Geometry check sheet. Reference: the model listing, model coordinates, mm. Round coordinates to 2 decimals unless told otherwise and drop trailing zeros. Order: outer loops, then holes, each group sorted by start corner. A loop starts at its lowest first (then second) coordinate and runs counter-clockwise, first axis right, second up.
Autodesk Inventor part; units mm, degrees
ref_plane "YZ Plane" through (0, 0, 0) normal (1, 0, 0) x (0, 1, 0)
ref_plane "XZ Plane" through (0, 0, 0) normal (0, 1, 0) x (-1, 0, 0)
ref_plane "XY Plane" through (0, 0, 0) normal (0, 0, 1) x (1, 0, 0)
sketch "スケッチ1" plane through (0, 0, 0) normal (0, 0, 1) x (1, 0, 0)
  line L0 (0, 0) -> (50, 0)
  line L1 (50, 0) -> (50, 115)
  line L2 (50, 115) -> (0, 115)
  line L3 (0, 115) -> (0, 0)
  circle A0 centre (25, 81.5) radius 9
  circle A1 centre (25, 33.5) radius 9
  line L4 (0, 0) -> (-18.7939, 6.8404)
  line L5 (-18.7939, 6.8404) -> (0, 80)
  line L6 (50, 0) -> (68.7939, 6.8404)
  line L7 (68.7939, 6.8404) -> (50, 80)
  line L8 (-18.7939, 6.8404) -> (68.7939, 6.8404)
  dimension "d0" = 50
  dimension "d1" = 115
  dimension "d2" = 18
  dimension "d3" = 18
  dimension "d5" = 48
  dimension "d8" = 33.5
  dimension "d27" = 20
  dimension "d28" = 20
  dimension "d34" = 80
  dimension "d35" = 80
  dimension "d36" = 20
  dimension "d37" = 20
extrude "押し出し1" add sketch "スケッチ1" along normal blind 2 contours L8 L5 L3 | L3 L2 L1 L8 | L1 L7 L8
sketch "スケッチ2" plane through (0, 0, 2) normal (0, 0, 1) x (1, 0, 0)
  line L0 (0, 115) -> (0, 0)
  line L1 (50, 80) -> (50, 115)
  line L2 (50, 115) -> (0, 115)
  point P0 (7.5, 107.5)
  point P1 (42.5, 107.5)
  point P2 (57.5, 15)
  point P3 (-7.5, 15)
  dimension "d15" = 7.5
  dimension "d16" = 7.5
  dimension "d17" = 7.5
  dimension "d18" = 7.5
  dimension "d31" = 7.5
  dimension "d32" = 7.5
  dimension "d40" = 15
  dimension "d41" = 15
hole "穴1" at (7.5, 107.5, 2) at (42.5, 107.5, 2) at (57.5, 15, 2) at (-7.5, 15, 2) direction (0, 0, -1) diameter 4 depth 8 tip angle 118
fillet "フィレット2" radius 7 6 edges at (50, 115, 1) (0, 115, 1) (0, 80, 1) (50, 80, 1) (-18.7939, 6.8404, 1) (68.7939, 6.8404, 1)
equation "\"d8\" = -0.5 * d5 + 0.5 * d1"
equation "\"d35\" = d34"
equation "\"d37\" = d36"
properties part number "TH22_AlBoard_roller_sub_sn" material "アルミニウム 6061-AHC"
(1) Sectioned sample at B-B, the plane x = 57.5. Record the cut outline in (y, z).
Returned:
outline: (6.84, 0) - (13, 0) - (13, 2) - (6.84, 2) - close; (17, 0) - (50.8, 0) - (50.8, 2) - (17, 2) - close
(2) Depth check by flat-ended pin: P1, Ø5, axis at x = -7.5, y = 15, coming from the -Z side; P2, Ø1, axis at y = 97.5, z = 1, coming from the -X side. Enter the tip coordinate at first touch or a pass-through.
Returned:
P1: stops at z = 0
P2: stops at x = 0
(3) Sectioned sample at D-D, the plane y = 103. Record the cut outline in (x, z).
Returned:
outline: (0, 0) - (50, 0) - (50, 2) - (0, 2) - close
(4) Sectioned sample at A-A, the plane z = 0.7. Record the cut outline in (x, y), and give its area (3 significant figures).
Returned:
outline: (-16.55, 15.58) arc R7 ccw to (-9.77, 6.84) - (59.77, 6.84) arc R7 ccw to (66.55, 15.58) - (50.22, 79.14) arc R7 cw to (50, 80.88) - (50, 108) arc R7 ccw to (43, 115) - (7, 115) arc R7 ccw to (0, 108) - (0, 80.88) arc R7 cw to (-0.22, 79.14) - close; hole circle Ø4 at (-7.5, 15); hole circle Ø4 at (7.5, 107.5); hole circle Ø18 at (25, 33.5); hole circle Ø18 at (25, 81.5); hole circle Ø4 at (42.5, 107.5); hole circle Ø4 at (57.5, 15)
area: 6,170 mm2
(5) Draft check along Y on faces 1 (the flat face through (24, 50, 0)), 2 (the flat face through (58.498, 46.918, 0.986)), 3 (the cylindrical face through (44.452, 107.934, 0.986)). Enter one of: released by +Y, released by -Y, zero draft, split by the parting line, or undercut.
Returned:
face 1: zero draft
face 2: released by +Y
face 3: undercut
(6) Material ranges on line 1 (X direction, y = 107.5, z = 0.65); line 2 (Y direction, x = 25, z = 0.6); line 3 (X direction, y = 15, z = 0.75), recorded low to high.
Returned:
line 1: x = 0 to 5.5, 9.5 to 40.5, 44.5 to 50
line 2: y = 6.84 to 24.5, 42.5 to 72.5, 90.5 to 115
line 3: x = -16.67 to -9.5, -5.5 to 55.5, 59.5 to 66.67
(7) Sectioned sample at C-C, the plane y = 30. Record the cut outline in (x, z).
Returned:
outline: (-12.84, 0) - (16.71, 0) - (16.71, 2) - (-12.84, 2) - close; (33.29, 0) - (62.84, 0) - (62.84, 2) - (33.29, 2) - close
